```python
from build123d import *


with BuildPart() as part:
    # Sketch1 → Revolve1 (revolve)
    with BuildSketch(Plane(origin=(0, 0, 0), x_dir=(0, 0, -1), z_dir=(1, 0, 0)), mode=Mode.PRIVATE) as revolve1_sk:
        with BuildLine():
            Line((0, 0), (0, 76.444627725))
            ThreePointArc((0, 76.444627725), (0.130798304, 76.879222907), (0.479738309, 77.169433247))
            Line((0.479738309, 77.169433247), (0.872854821, 77.336301306))
            ThreePointArc((0.872854821, 77.336301306), (1.6002, 78.4352), (0.872854821, 79.534098694))
            Line((0.872854821, 79.534098694), (0.479738309, 79.700966753))
            ThreePointArc((0.479738309, 79.700966753), (0.130798304, 79.991177093), (0, 80.425772275))
            Line((0, 80.425772275), (0, 83.439))
            Line((0, 83.439), (5.588, 83.439))
            Line((5.588, 83.439), (11.0998, 68.295453959))
            Line((11.0998, 68.295453959), (11.0998, 0))
            Line((11.0998, 0), (0, 0))
        make_face()
    revolve(revolve1_sk.sketch.rotate(Axis((0, 0, 0), (0, 0, -1)), 90), axis=Axis((0, 0, 0), (0, 0, -1)))


solid = part.part
```
Source: CAD feature listing. Evaluate the final solid. Frame: model axes, mm. Round coordinates to 2 decimals unless told otherwise and drop trailing zeros. Loops run counter-clockwise (first coordinate to the right, second up) from the corner with the lowest first, then second, coordinate; pieces in that order, holes last.
1. Ray query, L1, parallel to X at y = -45, z = -0.5; L2, parallel to Y at x = -48, z = -2.5; L3, parallel to Z at x = -25.5, y = 72. Return the intervals inside material, ascending.
2. Section query A-A on y = 0. Output: boundary loops of the cut face in (x, z), and give its area (3 significant figures).
3. Contact query for flat-ended pins moving along their axis: pin 1 (6 mm diameter, centred on x = -53, z = -5.5, fed in from +Y); pin 2 (5 mm diameter, centred on y = -6.5, z = -2, fed in from -X); pin 3 (6 mm diameter, centred on x = 32.5, z = -3, fed in from -Y). Output: stop coordinate, or through.
Answers below:
1. L1: x = -70.26 to -65.77, -62.7 to 62.7, 65.77 to 70.26
1. L2: y = -68.25 to 68.25
1. L3: z = -8.16 to 0
2. outline: (-83.44, -5.59) - (-68.3, -11.1) - (68.3, -11.1) - (83.44, -5.59) - (83.44, 0) - (80.43, 0) arc R0.79 ccw to (79.7, -0.48) - (79.53, -0.87) arc R1.19 cw to (77.34, -0.87) - (77.17, -0.48) arc R0.79 ccw to (76.44, 0) - (-76.44, 0) arc R0.79 ccw to (-77.17, -0.48) - (-77.34, -0.87) arc R1.19 cw to (-79.53, -0.87) - (-79.7, -0.48) arc R0.79 ccw to (-80.43, 0) - (-83.44, 0) - close
2. area: 1,760 mm2
3. pin 1: stops at y = 66.8
3. pin 2: stops at x = -83.34
3. pin 3: stops at y = -78.05
